```python
from build123d import *

# Parameters (mm, degrees)
BOSS_EXTRUDE1_DEPTH     = 101.6
CUT_EXTRUDE1_DEPTH      = 2.352318769
CUT_EXTRUDE1_DEPTH_BACK = 104.135020581
CUT_EXTRUDE2_DEPTH      = 1.679064128
CUT_EXTRUDE2_DEPTH_BACK = 102.6


with BuildPart() as part:
    # Sketch1 → Boss-Extrude1 (new body)
    with BuildSketch(Plane.XY):
        with BuildLine():
            Line((0, 79.375), (0, 180.975))
            ThreePointArc((0, 180.975), (11.836331312, 180.587518633), (23.621977637, 179.426733787))
            Line((23.621977637, 179.426733787), (10.360516507, 78.695935872))
            ThreePointArc((10.360516507, 78.695935872), (5.191373383, 79.205052032), (0, 79.375))
        make_face()
    extrude(amount=BOSS_EXTRUDE1_DEPTH)

    # Sketch5 → Cut-Extrude1 (cut, two sides)
    with BuildSketch(Plane(origin=(10.360516507, 78.695935872, 0), x_dir=(0, 0, -1), z_dir=(-0.130526192, -0.991444861, 0))) as cut_extrude1_sk:
        Polygon((-93.64987891, -3.175), (-84.12487891, -3.175), (-85.725, 0), (-92.04975782, 0), align=None)
        Polygon((-15.875, 0), (-17.47512109, -3.175), (-7.95012109, -3.175), (-9.55024218, 0), align=None)
    extrude(amount=CUT_EXTRUDE1_DEPTH, mode=Mode.SUBTRACT)
    extrude(cut_extrude1_sk.sketch, amount=-CUT_EXTRUDE1_DEPTH_BACK, mode=Mode.SUBTRACT)

    # Sketch6 → Cut-Extrude2 (cut, two sides)
    with BuildSketch(Plane(origin=(0, 79.375, 0), x_dir=(0, 0, -1), z_dir=(0, -1, 0))) as cut_extrude2_sk:
        Polygon((-84.1375, 3.059915209), (-93.6625, 3.059915209), (-92.06237891, 0), (-85.73762109, 0), align=None)
        Polygon((-15.86237891, 0), (-17.4625, 3.059915209), (-7.9375, 3.059915209), (-9.53762109, 0), align=None)
    extrude(amount=CUT_EXTRUDE2_DEPTH, mode=Mode.SUBTRACT)
    extrude(cut_extrude2_sk.sketch, amount=-CUT_EXTRUDE2_DEPTH_BACK, mode=Mode.SUBTRACT)


solid = part.part
```
Here's how the part is built. I have some questions about the finished solid (model axes, mm). A direction names the side the tool comes from. Give positions to 0.01 mm unless a question says otherwise; leave off trailing zeros. Write each loop counter-clockwise with the first axis right and the second up, starting at its lowest first coordinate (ties: lowest second). Pieces come first, ordered by that corner, then holes.
(1) On a 3-axis mill with a long thin cutter (end or side, diameter ignored), from which of +Z, -Z, +X, -X, +Y, -Y can I reach the whole of each face in a straight line? I mean faces 1 (the face through (3.06, 129, 89)), 2 (the face through (13.93, 130.14, 88.95)), 3 (the face through (17.084, 129.766, 50.311)). Say none if no direction works.
Output values:
face 1: +Y, -Y
face 2: none
face 3: +Z, -Z, +X, -Y
(2) Imagine slicing it at B-B, the plane x = 8.75. Write out the boundary of the cut face in (y, z).
Output values:
outline: (78.89, 0) - (180.76, 0) - (180.76, 101.6) - (78.89, 101.6) - (78.89, 92.87) - (90.79, 93.65) - (90.79, 84.12) - (78.89, 84.91) - (78.89, 16.69) - (90.79, 17.48) - (90.79, 7.95) - (78.89, 8.73) - close
(3) Imagine slicing it at D-D, the plane y = 171.5. Write out the boundary of the cut face in (x, z) (1 decimal), and give its area (3 significant figures).
Output values:
outline: (0, 0) - (22.6, 0) - (22.6, 9.6) - (19.4, 8) - (19.4, 17.5) - (22.6, 15.9) - (22.6, 85.7) - (19.4, 84.1) - (19.4, 93.6) - (22.6, 92) - (22.6, 101.6) - (0, 101.6) - (0, 92.1) - (3.1, 93.7) - (3.1, 84.1) - (0, 85.7) - (0, 15.9) - (3.1, 17.5) - (3.1, 7.9) - (0, 9.5) - close
area: 2,190 mm2
(4) Thinking about a two-plate mould opening in X: for faces 4 (the face through (0, 129, 5)), 5 (the face through (17.084, 129.766, 96.758)), 6 (the face through (15.484, 129.946, 8.739)), which applies, pulls with the +X half, pulls with the -X half, needs draft (parallel to the pull), parting line crosses it, or undercut?
Output values:
face 4: pulls with the -X half
face 5: pulls with the +X half
face 6: undercut
(5) Imagine slicing it at C-C, the plane z = 37. Write out the boundary of the cut face in (x, y) (3 decimals).
Output values:
outline: (0, 79.375) arc R79.375 cw to (10.361, 78.696) - (23.622, 179.427) arc R180.975 ccw to (0, 180.975) - close
(6) Will these pins go through, and if not, where does the flat tip stop? pin 1 (5 mm diameter, centred on y = 99.5, z = 43, fed in from +X); pin 2 (3 mm diameter, centred on x = 2.5, z = 17, fed in from +Y); pin 3 (3 mm diameter, centred on y = 154.5, z = 88, fed in from -X).
Output values:
pin 1: stops at x = 13.43
pin 2: stops at y = 180.97
pin 3: stops at x = 3.06
(7) Imagine slicing it at A-A, the plane y = 102. Write out the boundary of the cut face in (x, z) (1 decimal).
Output values:
outline: (0, 0) - (13.4, 0) - (13.4, 9.6) - (10.2, 8) - (10.2, 17.5) - (13.4, 15.9) - (13.4, 85.7) - (10.2, 84.1) - (10.2, 93.6) - (13.4, 92) - (13.4, 101.6) - (0, 101.6) - (0, 92.1) - (3.1, 93.7) - (3.1, 84.1) - (0, 85.7) - (0, 15.9) - (3.1, 17.5) - (3.1, 7.9) - (0, 9.5) - close
(8) If I drill on L1, parallel to Z at x = 2.25, y = 106.5; L2, parallel to Z at x = 3, y = 172; L3, parallel to Y at x = 3.25, z = 13.5, over which ranges is the centre line in solid material (lowest first)?
Output values:
L1: z = 0 to 8.36, 17.04 to 84.56, 93.24 to 101.6
L2: z = 0 to 7.97, 17.43 to 84.17, 93.63 to 101.6
L3: y = 79.31 to 180.95
